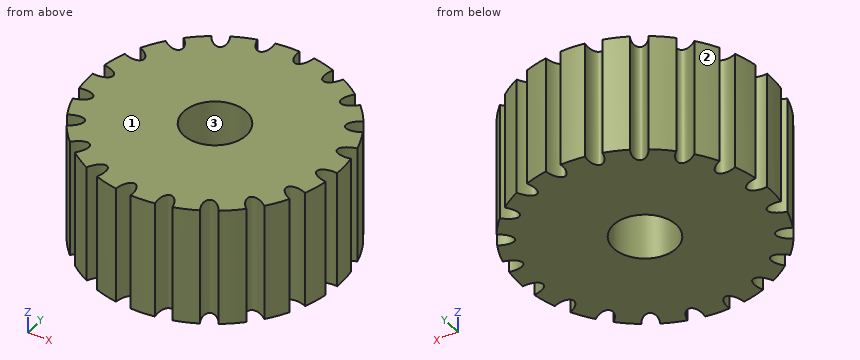
from build123d import *

# Parameters (mm, degrees)
SKETCH_1_R               = 15.91549431
EXTRUDE_2_DEPTH          = 15
SKETCH_2_R               = 4
CUT_EXTRUDE_1_DEPTH      = 15
SKETCH_3_RX              = 2
SKETCH_3_RY              = 1
CUT_EXTRUDE_2_DEPTH      = 15
PATTERN_CIRCULAR_1_COUNT = 20


with BuildPart() as part:
    # Эскиз1 → Бобышка-Вытянуть2 (new body)
    with BuildSketch(Plane.XY):
        Circle(SKETCH_1_R)
    extrude(amount=EXTRUDE_2_DEPTH)

    # Эскиз2 → Вырез-Вытянуть1 (cut)
    with BuildSketch(Plane.XY.offset(15)):
        Circle(SKETCH_2_R)
    extrude(amount=-CUT_EXTRUDE_1_DEPTH, mode=Mode.SUBTRACT)

    # Эскиз3 → Вырез-Вытянуть2 (cut)
    with BuildSketch(Plane.XY.offset(15)):
        with Locations(Location((13.72327338, 8.060690222), (0, 0, 30.428856936))):
            Ellipse(SKETCH_3_RX, SKETCH_3_RY)
    cut_extrude_2 = extrude(amount=-CUT_EXTRUDE_2_DEPTH, mode=Mode.SUBTRACT)

    # Круговой массив1: Вырез-Вытянуть2 ×20 about axis
    pattern_circular_1_axis = Axis((0, 0, 15), (0, 0, 1))
    for i in range(1, PATTERN_CIRCULAR_1_COUNT):
        add(cut_extrude_2.rotate(pattern_circular_1_axis, i * 360 / PATTERN_CIRCULAR_1_COUNT), mode=Mode.SUBTRACT)


solid = part.part
Could you check a few things on this model? Use its own coordinates, in mm. Face numbers are marked on the shaded views. Coordinates: 2 decimals unless noted, no trailing zeros. Write each loop counter-clockwise with the first axis right and the second up, starting at its lowest first coordinate (ties: lowest second). Pieces come first, ordered by that corner, then holes. Notation, with made-up numbers: (21.25, -13.75) - (71.25, -13.75) arc R16 cw to (71.25, -2.75) - close; hole circle Ø3 at (39, 12.25). An arc over 180 degrees is marked (long way). Write item = value, one per line.
1) We'd pull the mould along Y, two halves only. Please class the marked faces 1, 2 and 3: +Y half, -Y half, draft (parallel to the pull), parting line (faces both ways), or undercut.
Result set:
face_1 = draft
face_2 = +Y half
face_3 = undercut
2) Please list where these lines run through material, in increasing order: line 1 (Y direction, x = 0, z = 4.75); line 2 (X direction, y = 13, z = 4.25); line 3 (X direction, y = -14, z = 6.75). Write a range as [from, to].
Result set:
line_1 = [-15.92, -4], [4, 15.92]
line_2 = [-9.18, -8.79], [-6.75, 5.3], [6.44, 9.18]
line_3 = [-7.57, -7.19], [-5.17, -1.8], [-1.03, 2.54], [3.8, 7.07]
3) Will these pins go through, and if not, where does the flat tip stop? pin 1 Ø3 at (y, z) = (-9.5, 6.5) entering from -X; pin 2 Ø1 at (x, y) = (1.5, -9.5) entering from -Z; pin 3 Ø4 at (y, z) = (-4, 10.5) entering from +X; pin 4 Ø4 at (y, z) = (4, 9) entering from -X.
Result set:
pin_1 = -13.19
pin_2 = 0
pin_3 = 15.71
pin_4 = -15.71
4) Suppose I cut it at A-A on x = 0. Please give me the cut outline in (y, z), plus the area to 3 significant figures.
Result set:
outline = (-15.92, 0) - (-4, 0) - (-4, 15) - (-15.92, 15) - close; (4, 0) - (15.92, 0) - (15.92, 15) - (4, 15) - close
area = 357 mm2
